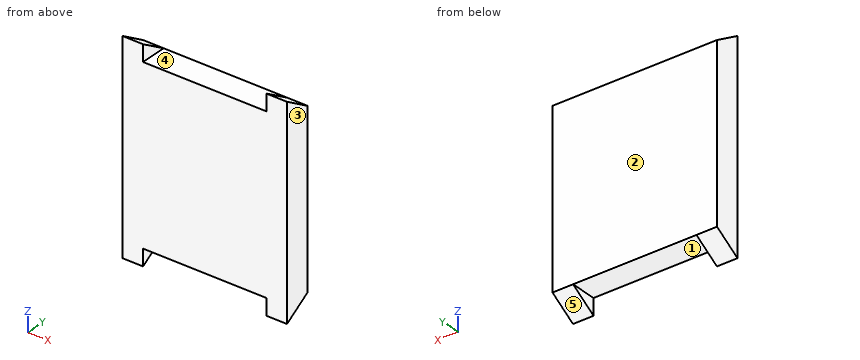
from build123d import *

# Parameters (mm, degrees)
SKETCH1_W           = 800
SKETCH1_H           = 1000
BOSS_EXTRUDE1_DEPTH = 129
CUT_EXTRUDE1_DEPTH  = 800
SKETCH17_W          = 600
SKETCH17_H          = 151.792621691
CUT_EXTRUDE2_DEPTH  = 275
SKETCH25_W          = 600
SKETCH25_H          = 129
CUT_EXTRUDE4_DEPTH  = 80
CUT_EXTRUDE5_DEPTH  = 100
CUT_EXTRUDE6_DEPTH  = 100
BOSS_EXTRUDE4_DEPTH = 600


with BuildPart() as part:
    # Sketch1 → Boss-Extrude1 (new body)
    with BuildSketch(Plane(origin=(0, 0, 0), x_dir=(1, 0, 0), z_dir=(0, 1, 0))):
        Rectangle(SKETCH1_W, SKETCH1_H)
    extrude(amount=BOSS_EXTRUDE1_DEPTH)

    # Sketch2 → Cut-Extrude1 (cut)
    with BuildSketch(Plane.ZY.offset(400)):
        Polygon((420, 129), (500, 0), (500, 129), align=None)
    extrude(amount=-CUT_EXTRUDE1_DEPTH, mode=Mode.SUBTRACT)

    # Sketch17 → Cut-Extrude2 (cut)
    with BuildSketch(Plane(origin=(0, 223.948613341, 361.117139013), x_dir=(1, 0, 0), z_dir=(0, 0.5270348394308224, 0.849843678582201))):
        with Locations((0, -187.62110887)):
            Rectangle(SKETCH17_W, SKETCH17_H)
    extrude(amount=-CUT_EXTRUDE2_DEPTH, mode=Mode.SUBTRACT)

    # Sketch25 → Cut-Extrude4 (cut)
    with BuildSketch(Plane(origin=(0, 0, -500), x_dir=(-1, 0, 0), z_dir=(0, 0, -1))):
        with Locations((0, 64.5)):
            Rectangle(SKETCH25_W, SKETCH25_H)
    extrude(amount=-CUT_EXTRUDE4_DEPTH, mode=Mode.SUBTRACT)

    # Sketch28 → Cut-Extrude5 (cut)
    with BuildSketch(Plane(origin=(-300, 0, 0), x_dir=(0, 0, -1), z_dir=(1, 0, 0))):
        Polygon((420, 129), (500, 129), (500, 0), align=None)
    extrude(amount=-CUT_EXTRUDE5_DEPTH, mode=Mode.SUBTRACT)

    # Sketch29 → Cut-Extrude6 (cut)
    with BuildSketch(Plane.ZY.offset(-300)):
        Polygon((-420, 129), (-500, 129), (-500, 0), align=None)
    extrude(amount=-CUT_EXTRUDE6_DEPTH, mode=Mode.SUBTRACT)

    # Sketch31 → Boss-Extrude4 (add)
    with BuildSketch(Plane.ZY.offset(-300)):
        Polygon((420, 129), (420, 0), (211.9875, 0), align=None)
    extrude(amount=BOSS_EXTRUDE4_DEPTH)


solid = part.part
For this review, take the finished solid that the model builds, in its own axes (mm). Face numbers are marked on the shaded views. A direction names the side the tool comes from. Round coordinates to 2 decimals unless told otherwise and drop trailing zeros. Order: outer loops, then holes, each group sorted by start corner. A loop starts at its lowest first (then second) coordinate and runs counter-clockwise, first axis right, second up. Notation, with made-up numbers: M 0.5,46.25 L 23.5,46.25 A18 cw 23.5,77.25 Z; hole C 86,56.5 d4. An arc over 180 degrees is marked long. Use a Markdown table: item, result. Add a question column.
Item 1: Tool access review of the marked faces 1 and 2: name each direction out of +Z, -Z, +X, -X, +Y, -Y from which nothing blocks a thin tool from reaching the whole face with its end or side.
Item 2: Insertion check: pin 1 (8 mm diameter, centred on x = -127, y = 78, fed in from -Z); pin 2 (5 mm diameter, centred on x = -219.5, y = 41, fed in from +Z). Each pin has a flat end and moves straight along its axis. Give the tip position at first contact, or say it passes through.
Item 3: Mouldability with a two-part tool opening along X and no side actions: class the marked faces 3, 4 and 5 as released by +X, released by -X, zero draft, split by the parting line, or undercut.
Item 4: Add section A-A, the plane y = 73. Give the boundary of the cut face in (x, z).
Item 5: Add section C-C, the plane x = 313. Give the boundary of the cut face in (y, z), then the cut area to 3 significant figures.
Item 6: To check wall thickness, follow line 1 along Z through (x, y) = (-100.5, 54.5). State the ranges of the line that lie inside material, in increasing order.
Item 7: Add section B-B, the plane x = 193.5. Give the boundary of the cut face in (y, z).
Geometry results:
| question | item | result |
|---|---|---|
| 1 | face 1 | -Z, +Y, -Y |
| 1 | face 2 | +Z, -Z, +X, -X, +Y |
| 2 | pin 1 | stops at z = -420 |
| 2 | pin 2 | stops at z = 420 |
| 3 | face 3 | released by +X |
| 3 | face 4 | undercut |
| 3 | face 5 | zero draft |
| 4 | outline | M -400,-454.73 L -300,-454.73 L -300,-420 L 300,-420 L 300,-454.73 L 400,-454.73 L 400,454.73 L 300,454.73 L 300,420 L -300,420 L -300,454.73 L -400,454.73 Z |
| 5 | outline | M 0,-500 L 129,-420 L 129,420 L 0,500 Z |
| 5 | area | 119,000 mm² |
| 6 | line 1 | z = -420 to 420 |
| 7 | outline | M 0,-420 L 129,-420 L 129,420 L 0,420 Z |
